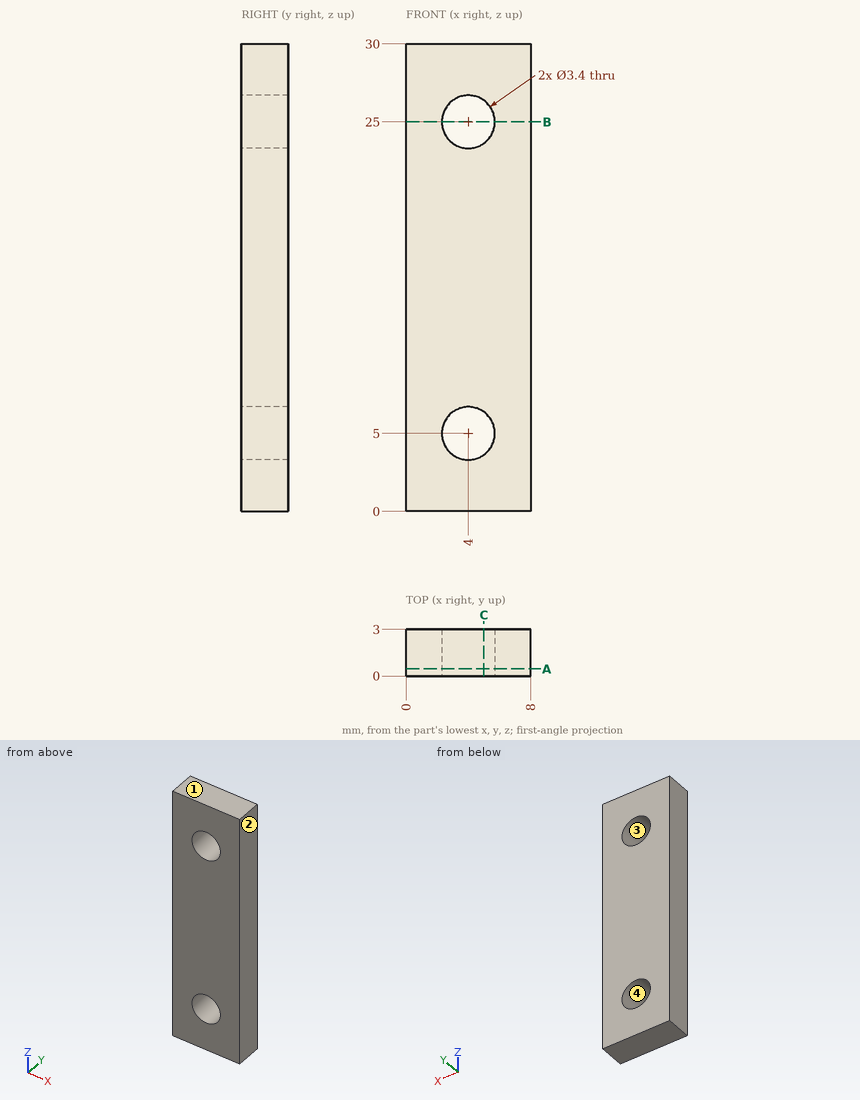
The figure shows three views and two pictorial views of one solid part (mm, origin at its lowest corner). Answer the questions. Coordinates: 2 decimals unless noted, no trailing zeros. Loops run counter-clockwise (first coordinate to the right, second up) from the corner with the lowest first, then second, coordinate; pieces in that order, holes last. Notation, with made-up numbers: (-20.75, 3.25) -> (26.25, 3.25) arc R19 ccw to (26.25, 28.25) -> close; hole circle Ø10 at (80, 6). An arc over 180 degrees is marked (long way). Use one line per item in the form item = value. Start each with the question number.
Item 1: The part is cut by section B-B on z = 25. Determine the outline of the cut face in (x, y).
Item 2: The part is cut by section C-C on x = 5. Determine the outline of the cut face in (y, z), then the cut area to 3 significant figures.
Item 3: The mould has two halves that part along X. Classify the marked faces 1, 2, 3 and 4: released by +X, released by -X, zero draft, split by the parting line, or undercut.
Item 4: Consider L1, parallel to Z at x = 4, y = 0.7; L2, parallel to Z at x = 5.5, y = 2; L3, parallel to X at y = 1.75, z = 5. Determine where each line is inside the solid, lowest interval first. Write a range as [from, to].
Item 5: The part is cut by section A-A on y = 0.45. Determine the outline of the cut face in (x, z).
Answer key:
q1.outline = (0, 0) -> (2.3, 0) -> (2.3, 3) -> (0, 3) -> close; (5.7, 0) -> (8, 0) -> (8, 3) -> (5.7, 3) -> close
q2.outline = (0, 0) -> (3, 0) -> (3, 3.63) -> (0, 3.63) -> close; (0, 6.37) -> (3, 6.37) -> (3, 23.63) -> (0, 23.63) -> close; (0, 26.37) -> (3, 26.37) -> (3, 30) -> (0, 30) -> close
q2.area = 73.5 mm2
q3.face_1 = zero draft
q3.face_2 = released by +X
q3.face_3 = undercut
q3.face_4 = undercut
q4.L1 = [0, 3.3], [6.7, 23.3], [26.7, 30]
q4.L2 = [0, 4.2], [5.8, 24.2], [25.8, 30]
q4.L3 = [0, 2.3], [5.7, 8]
q5.outline = (0, 0) -> (8, 0) -> (8, 30) -> (0, 30) -> close; hole circle Ø3.4 at (4, 5); hole circle Ø3.4 at (4, 25)
